Study the drawing (mm; zero at the part's minimum x, y, z) and answer. A direction names the side the tool comes from. Give positions to 0.01 mm unless a question says otherwise; leave off trailing zeros. Order: outer loops, then holes, each group sorted by start corner. A loop starts at its lowest first (then second) coordinate and runs counter-clockwise, first axis right, second up.
Item 1: The mould has two halves that part along X. Classify the marked faces 4, 5 and 6: +X half, -X half, draft (parallel to the pull), parting line (faces both ways), or undercut.
Item 2: A cutting plane is placed at C-C (x = 14.25). Write down the section's boundary in (y, z).
Item 3: Which of the six approach directions +Z, -Z, +X, -X, +Y, -Y give full straight-line access (tool end or side, diameter ignored) to the marked faces 1, 2 and 3?
Item 4: A cutting plane is placed at A-A (y = 18.75). Write down the section's boundary in (x, z) (1 decimal).
Item 5: A cutting plane is placed at D-D (y = 2.5). Write down the section's boundary in (x, z) (1 decimal).
Item 6: Find the intervals of material crossed by line 1 along Y through (x, z) = (9, 2.25); line 2 along X through (y, z) = (20.5, 9.25) (1 decimal); line 3 along X through (y, z) = (15.5, 2), in increasing order.
Item 7: Given pin 1 Ø4.5 at (y, z) = (15.5, 8.5) entering from -X (1 decimal); pin 2 Ø2 at (x, y) = (19.5, 14) entering from +Z (1 decimal); pin 3 Ø7.5 at (y, z) = (14.41, 8.06) entering from +X (1 decimal), each flat-ended and moving along its own axis, determine where each tip first touches the part or whether it passes through.
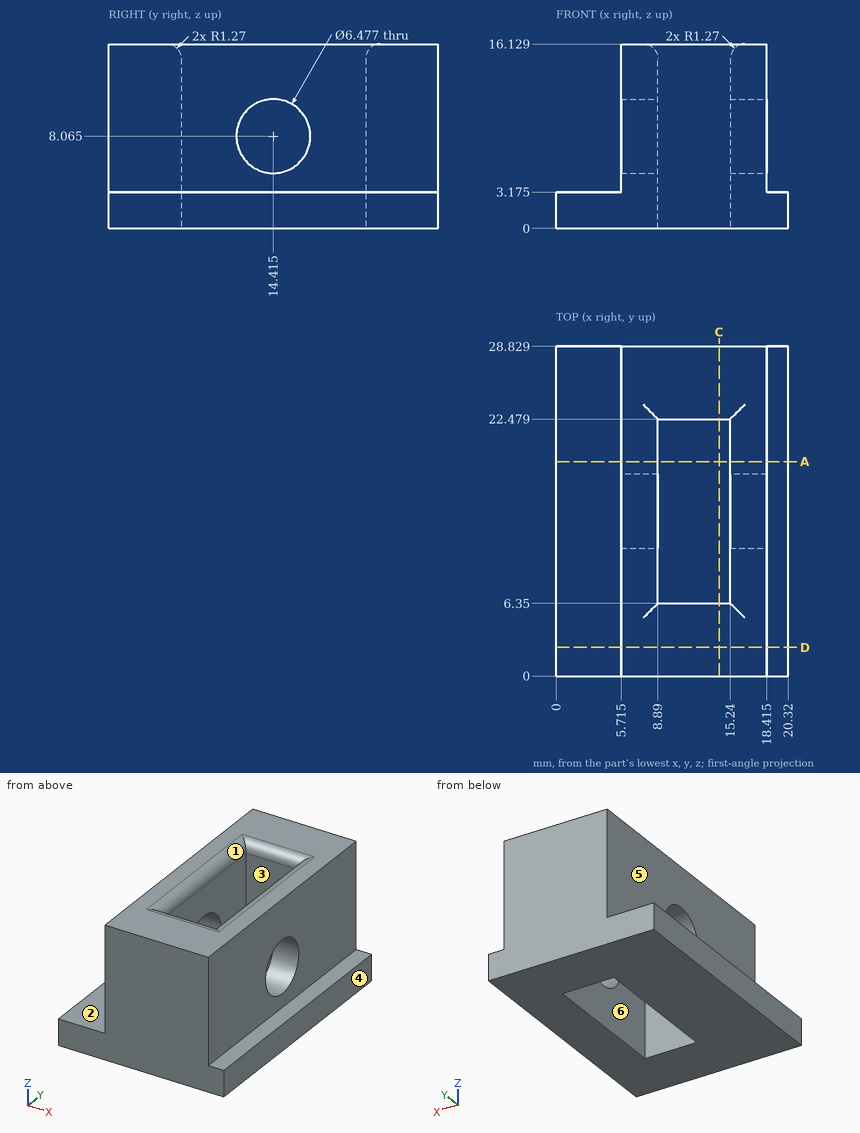
Response values:
1. face 4: +X half
1. face 5: -X half
1. face 6: undercut
2. outline: (0, 0) - (6.35, 0) - (6.35, 14.86) arc R1.27 ccw to (5.08, 16.13) - (0, 16.13) - close; (22.48, 0) - (28.83, 0) - (28.83, 16.13) - (23.75, 16.13) arc R1.27 ccw to (22.48, 14.86) - close
3. face 1: +Z
3. face 2: +Z, -X, +Y, -Y
3. face 3: +Z, -Z
4. outline: (0, 0) - (8.9, 0) - (8.9, 14.9) arc R1.3 ccw to (7.6, 16.1) - (5.7, 16.1) - (5.7, 3.2) - (0, 3.2) - close; (15.2, 0) - (20.3, 0) - (20.3, 3.2) - (18.4, 3.2) - (18.4, 16.1) - (16.5, 16.1) arc R1.3 ccw to (15.2, 14.9) - close
5. outline: (0, 0) - (20.3, 0) - (20.3, 3.2) - (18.4, 3.2) - (18.4, 16.1) - (5.7, 16.1) - (5.7, 3.2) - (0, 3.2) - close
6. line 1: y = 0 to 6.35, 22.48 to 28.83
6. line 2: x = 5.7 to 8.9, 15.2 to 18.4
6. line 3: x = 0 to 8.89, 15.24 to 20.32
7. pin 1: stops at x = 5.7
7. pin 2: stops at z = 3.2
7. pin 3: stops at x = 18.4
